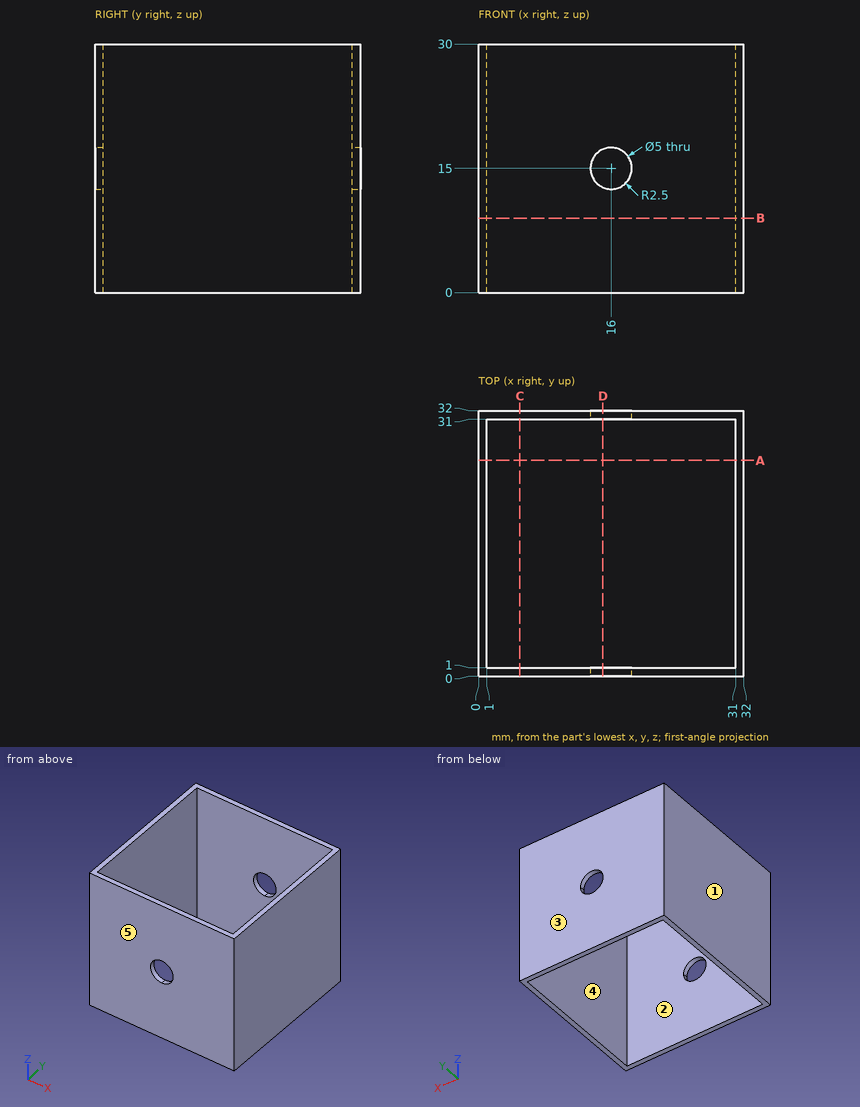
Part print with two shaded views. Sizes in mm from the minimum x, y, z corner. A direction names the side the tool comes from. Round coordinates to 2 decimals unless told otherwise and drop trailing zeros. Order: outer loops, then holes, each group sorted by start corner. A loop starts at its lowest first (then second) coordinate and runs counter-clockwise, first axis right, second up. Notation, with made-up numbers: (-6, -14.5) -> (32, -14.5) arc R4 cw to (32, -8.5) -> close; hole circle Ø8 at (-11, 73). An arc over 180 degrees is marked (long way). One line per question, with ' | ' between items.
Q1. Slice it at B-B (z = 9). Write the cut outline in (x, y).
Completed:
outline: (0, 0) -> (32, 0) -> (32, 32) -> (0, 32) -> close; hole (1, 1) -> (31, 1) -> (31, 31) -> (1, 31) -> close
Q2. Probe probe 1 along X at (y, z) = (2, 25); probe 2 along X at (y, z) = (31.75, 15); probe 3 along Z at (x, y) = (16, 31.6). List the from-to ranges inside material, lowest first.
Completed:
probe 1: x = 0 to 1, 31 to 32 | probe 2: x = 0 to 13.5, 18.5 to 32 | probe 3: z = 0 to 12.5, 17.5 to 30
Q3. Drop a flat-ended pin along its axis: pin 1 (4.5 mm diameter, centred on x = 16, z = 15, fed in from -Y). Give the stop position or say it passes through.
Completed:
pin 1: passes through
Q4. Which spindle directions (+Z, -Z, +X, -X, +Y, -Y) get a long thin tool onto all of the face, cutting with end or side? Do the marked faces 4 and 5. Say none if no direction does.
Completed:
face 4: +Z, -Z | face 5: +Z, -Z, +X, -X, -Y
Q5. Slice it at A-A (y = 26). Write the cut outline in (x, z).
Completed:
outline: (0, 0) -> (1, 0) -> (1, 30) -> (0, 30) -> close; (31, 0) -> (32, 0) -> (32, 30) -> (31, 30) -> close
Q6. Two-plate mould, pull along X, no slides. Class the marked faces 1, 2 and 3: released by +X, released by -X, zero draft, split by the parting line, or undercut.
Completed:
face 1: released by -X | face 2: undercut | face 3: zero draft
Q7. Slice it at D-D (x = 15). Write the cut outline in (y, z).
Completed:
outline: (0, 0) -> (1, 0) -> (1, 12.71) -> (0, 12.71) -> close; (0, 17.29) -> (1, 17.29) -> (1, 30) -> (0, 30) -> close; (31, 0) -> (32, 0) -> (32, 12.71) -> (31, 12.71) -> close; (31, 17.29) -> (32, 17.29) -> (32, 30) -> (31, 30) -> close
